```python
from build123d import *

# Parameters (mm, degrees)
BOSS_EXTRUDE1_DEPTH = 125
SKETCH2_W           = 35
SKETCH2_H           = 75
SKETCH2_W_2         = 15
CUT_EXTRUDE1_DEPTH  = 100
SKETCH3_R           = 8.75
BOSS_EXTRUDE2_DEPTH = 75
SKETCH4_W           = 200
SKETCH4_H           = 30
CUT_EXTRUDE2_DEPTH  = 230.401394939
FILLET1_R           = 10
SKETCH6_R           = 6.25
BOSS_EXTRUDE3_DEPTH = 22.5
SKETCH7_W           = 20
SKETCH7_H           = 5
BOSS_EXTRUDE4_DEPTH = 40
FILLET2_R           = 7.5


with BuildPart() as part:
    # Sketch1 → Boss-Extrude1 (new body)
    with BuildSketch(Plane.XY):
        with BuildLine():
            Line((-175, 15), (175, 15))
            ThreePointArc((175, 15), (190, 0), (175, -15))
            Line((175, -15), (-175, -15))
            ThreePointArc((-175, -15), (-190, 0), (-175, 15))
        make_face()
    extrude(amount=BOSS_EXTRUDE1_DEPTH)

    # Sketch2 → Cut-Extrude1 (cut)
    with BuildSketch(Plane(origin=(0, 15, 0), x_dir=(1, 0, 0), z_dir=(0, 1, 0))):
        with Locations((-157.5, -62.5)):
            Rectangle(SKETCH2_W, SKETCH2_H)
        with Locations((-182.5, -62.5)):
            Rectangle(SKETCH2_W_2, SKETCH2_H)
        with Locations((182.5, -62.5)):
            Rectangle(SKETCH2_W_2, SKETCH2_H)
        with Locations((157.5, -62.5)):
            Rectangle(SKETCH2_W, SKETCH2_H)
    extrude(amount=-CUT_EXTRUDE1_DEPTH, mode=Mode.SUBTRACT)

    # Sketch3 → Boss-Extrude2 (add)
    with BuildSketch(Plane.XY.offset(25)):
        with Locations(Location((-175, 0, 0), (0, 0, 180))):
            Circle(SKETCH3_R)
        with Locations(Location((175, 0, 0), (0, 0, 180))):
            Circle(SKETCH3_R)
    extrude(amount=BOSS_EXTRUDE2_DEPTH)

    # Sketch4 → Cut-Extrude2 (cut, through all)
    with BuildSketch(Plane(origin=(0, 15, 0), x_dir=(1, 0, 0), z_dir=(0, 1, 0))):
        with Locations((0, -15)):
            Rectangle(SKETCH4_W, SKETCH4_H)
        with Locations((0, -110)):
            Rectangle(SKETCH4_W, SKETCH4_H)
    extrude(amount=-CUT_EXTRUDE2_DEPTH, mode=Mode.SUBTRACT)

    # Fillet1
    fillet1_edges = [part.edges().sort_by_distance(p)[0] for p in [
        (-100, 0, 0),
        (100, 0, 0),
        (100, 0, 125),
        (-100, 0, 125),
    ]]
    fillet(fillet1_edges, radius=FILLET1_R)



with BuildPart() as body_2:
    # Sketch6 → Boss-Extrude3 (new, symmetric)
    with BuildSketch(Plane.XY.offset(62.5)):
        with Locations(Location((-30, 30, 0), (0, 0, 180))):
            Circle(SKETCH6_R)
    extrude(amount=BOSS_EXTRUDE3_DEPTH, both=True)


with BuildPart() as part_1:
    add(part.part)

    add(body_2.part)  # Boss-Extrude4 merges body 2
    # Sketch7 → Boss-Extrude4 (add)
    with BuildSketch(Plane(origin=(0, 0, 0), x_dir=(1, 0, 0), z_dir=(0, 1, 0))):
        with Locations((-30.433316443, -87.433842939)):
            Rectangle(SKETCH7_W, SKETCH7_H)
        with Locations((-30.433316443, -37.333363873)):
            Rectangle(SKETCH7_W, SKETCH7_H)
    extrude(amount=BOSS_EXTRUDE4_DEPTH)

    # Fillet2
    fillet2_edges = [part_1.edges().sort_by_distance(p)[0] for p in [
        (-20.433316443, 40, 87.433842939),
        (-40.433316443, 40, 87.433842939),
        (-40.433316443, 40, 37.333363873),
        (-20.433316443, 40, 37.333363873),
    ]]
    fillet(fillet2_edges, radius=FILLET2_R)


solid = part_1.part
```
Input: part model. Units: mm. Frame: model coordinates. A direction names the side the tool comes from. Coordinates: 2 decimals unless noted, no trailing zeros. Write each loop counter-clockwise with the first axis right and the second up, starting at its lowest first coordinate (ties: lowest second). Pieces come first, ordered by that corner, then holes. Notation, with made-up numbers: (-37, -13.75) -> (-24, -13.75) arc R24 cw to (-24, 24.25) -> close; hole circle Ø11 at (59.25, 12.5). An arc over 180 degrees is marked (long way). Answer as a JSON object with one key per item and string values.
1. Material intervals for line 1 (X direction, y = -1, z = 41); line 2 (X direction, y = 5, z = 97); line 3 (X direction, y = -9, z = 27), sorted ascending. Write a range as from..to.
Result set:
{"line 1": "x = -183.69..-166.31, -140..140, 166.31..183.69", "line 2": "x = -182.18..-167.82, -140..-100, 100..140, 167.82..182.18", "line 3": "x = -140..-100, 100..140"}
2. Section A-A on z = 44. Return the cut outline in (x, y).
Result set:
{"outline": "circle Ø17.5 at (-175, 0); (-140, -15) -> (140, -15) -> (140, 15) -> (-140, 15) -> close; circle Ø12.5 at (-30, 30); circle Ø17.5 at (175, 0)"}
3. Mould query, pull axis X, two halves, no side actions, for faces 1 (the face through (-100, 0, 105)), 2 (the face through (-22.57, 37.74, 37.3)), 3 (the face through (151, 0, 0)), 4 (the face through (140, 0, 63)). Classes: released by +X, released by -X, zero draft, split by the parting line, or undercut.
Result set:
{"face 1": "undercut", "face 2": "released by +X", "face 3": "zero draft", "face 4": "undercut"}
4. Section B-B on y = 0. Count the separate pieces of the cut face and the enclosed holes in it, then the cut area to 3 significant figures.
Result set:
{"separate pieces": "1", "enclosed holes": "2", "area": "30,500 mm2"}
5. Access query for faces 5 (the face through (102.85, -0.21, 3.01)), 6 (the face through (103.01, -0.21, 122.15)), 7 (the face through (-140, 0, 63)). Directions: +Z, -Z, +X, -X, +Y, -Y. A direction counts if a zero-diameter tool reaches every point of the face in a straight line with its end or side. Return the directions, or none.
Result set:
{"face 5": "-Z, +Y, -Y", "face 6": "+Z, +Y, -Y", "face 7": "+Y, -Y"}
6. Section C-C on x = 66. Return the cut outline in (y, z), then the cut area to 3 significant figures.
Result set:
{"outline": "(-15, 30) -> (15, 30) -> (15, 95) -> (-15, 95) -> close", "area": "1,950 mm2"}
7. First-contact query: P1, Ø10, axis at y = -3.5, z = 37.5, coming from the -X side; P2, Ø6, axis at y = 2, z = 102, coming from the +X side; P3, Ø1.5, axis at x = -61.5, z = 80, coming from the +Y side; P4, Ø5.5, axis at y = 26.5, z = 87, coming from the +X side. Flat tips, straight axial feed; report the tip coordinate or a pass-through.
Result set:
{"P1": "stops at x = -183.75", "P2": "stops at x = 190", "P3": "stops at y = 15", "P4": "stops at x = -20.43"}
